Source: CAD feature listing. Evaluate the final solid. Frame: model axes, mm. Face numbers are marked on the shaded views. A direction names the side the tool comes from. Round coordinates to 2 decimals unless told otherwise and drop trailing zeros. Write each loop counter-clockwise with the first axis right and the second up, starting at its lowest first coordinate (ties: lowest second). Pieces come first, ordered by that corner, then holes. Notation, with made-up numbers: M -31.5,3.25 L 6.5,3.25 A13 cw 6.5,24.25 Z; hole C 8.5,25 d1. An arc over 180 degrees is marked long. Use a Markdown table: item, result.
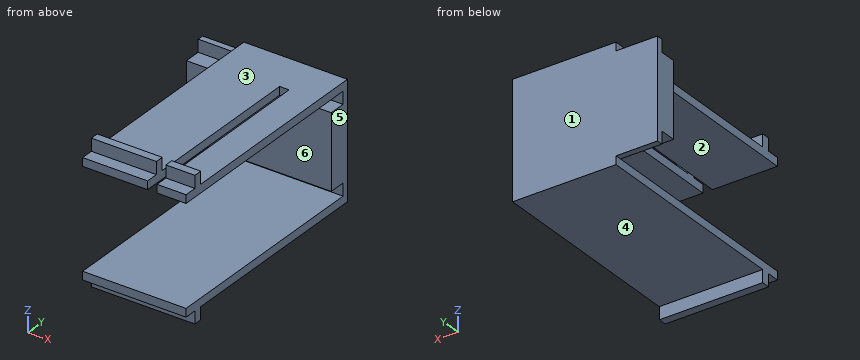
```python
from build123d import *

# Parameters (mm, degrees)
SKETCH1_W           = 25
SKETCH1_H           = 55
BOSS_EXTRUDE1_DEPTH = 2
SKETCH2_W           = 35
SKETCH2_H           = 1.5
BOSS_EXTRUDE2_DEPTH = 24
SKETCH3_W           = 25
SKETCH3_H           = 55
BOSS_EXTRUDE3_DEPTH = 2
SKETCH4_W           = 35
SKETCH4_H           = 18
BOSS_EXTRUDE4_DEPTH = 4
SKETCH5_W           = 2.3
SKETCH5_H           = 45
CUT_EXTRUDE1_DEPTH  = 2
SKETCH6_W           = 15.7
SKETCH6_H           = 2
SKETCH6_W_2         = 7
BOSS_EXTRUDE5_DEPTH = 3
SKETCH7_W           = 25
SKETCH7_H           = 2
BOSS_EXTRUDE6_DEPTH = 3


with BuildPart() as part:
    # Sketch1 → Boss-Extrude1 (new body)
    with BuildSketch(Plane.XY):
        Rectangle(SKETCH1_W, SKETCH1_H)
    extrude(amount=BOSS_EXTRUDE1_DEPTH)

    # Sketch2 → Boss-Extrude2 (add)
    with BuildSketch(Plane(origin=(0, 0, 0), x_dir=(-1, 0, 0), z_dir=(0, 0, -1))):
        with Locations((5, 26.75)):
            Rectangle(SKETCH2_W, SKETCH2_H)
    extrude(amount=BOSS_EXTRUDE2_DEPTH)

    # Sketch3 → Boss-Extrude3 (add)
    with BuildSketch(Plane(origin=(0, 0, -24), x_dir=(-1, 0, 0), z_dir=(0, 0, -1))):
        Rectangle(SKETCH3_W, SKETCH3_H)
    extrude(amount=BOSS_EXTRUDE3_DEPTH)

    # Sketch4 → Boss-Extrude4 (add)
    with BuildSketch(Plane.XZ.offset(-26)):
        with Locations((-5, -12)):
            Rectangle(SKETCH4_W, SKETCH4_H)
    extrude(amount=BOSS_EXTRUDE4_DEPTH)

    # Sketch5 → Cut-Extrude1 (cut)
    with BuildSketch(Plane.XY.offset(2)):
        with Locations((4.35, -5)):
            Rectangle(SKETCH5_W, SKETCH5_H)
    extrude(amount=-CUT_EXTRUDE1_DEPTH, mode=Mode.SUBTRACT)

    # Sketch6 → Boss-Extrude5 (add)
    with BuildSketch(Plane.XY.offset(2)):
        with Locations((-4.65, -23.5)):
            Rectangle(SKETCH6_W, SKETCH6_H)
        with Locations((9, -23.5)):
            Rectangle(SKETCH6_W_2, SKETCH6_H)
    extrude(amount=BOSS_EXTRUDE5_DEPTH)

    # Sketch7 → Boss-Extrude6 (add)
    with BuildSketch(Plane(origin=(0, 0, -26), x_dir=(-1, 0, 0), z_dir=(0, 0, -1))):
        with Locations((0, -23.5)):
            Rectangle(SKETCH7_W, SKETCH7_H)
    extrude(amount=BOSS_EXTRUDE6_DEPTH)


solid = part.part
```
Q1. Section B-B on x = -14. Return loops of the section in (y, z).
Results are:
| item | result |
|---|---|
| outline | M 22,-21 L 26,-21 L 26,-24 L 27.5,-24 L 27.5,0 L 26,0 L 26,-3 L 22,-3 Z |
Q2. Line query: L1, parallel to Z at x = -11.5, y = -6.5; L2, parallel to Z at x = -4, y = 23; L3, parallel to Z at x = -9.5, y = -23. Output: solid intervals per line, ascending.
Results are:
| item | result |
|---|---|
| L1 | -26 to -24, 0 to 2 |
| L2 | -26 to -24, -21 to -3, 0 to 2 |
| L3 | -29 to -24, 0 to 5 |
Q3. First-contact query: pin 1 Ø3 at (x, y) = (-12.5, 24) entering from -Z; pin 2 Ø3 at (x, z) = (-4, -20) entering from -Y; pin 3 Ø5.5 at (y, z) = (12.5, 3.5) entering from -X. Flat tips, straight axial feed; report the tip coordinate or a pass-through.
Results are:
| item | result |
|---|---|
| pin 1 | z = -26 |
| pin 2 | y = 22 |
| pin 3 | x = -12.5 |
Q4. Reachability of the marked faces 4, 5 and 6 from +Z, -Z, +X, -X, +Y, -Y: full face, straight path, thin tool, end or side. Return the list, or none.
Results are:
| item | result |
|---|---|
| face 4 | -Z, +X, -X, +Y |
| face 5 | +Z, -Z, +X, +Y, -Y |
| face 6 | +X, -X, -Y |
Q5. Section C-C on y = 24. Return loops of the section in (x, z), plus the area to 3 significant figures.
Results are:
| item | result |
|---|---|
| outline | M -22.5,-21 L 12.5,-21 L 12.5,-3 L -22.5,-3 Z; M -12.5,-26 L 12.5,-26 L 12.5,-24 L -12.5,-24 Z; M -12.5,0 L 12.5,0 L 12.5,2 L -12.5,2 Z |
| area | 730 mm^2 |
Q6. Section D-D on x = 10. Return loops of the section in (y, z), plus the area to 3 significant figures.
Results are:
| item | result |
|---|---|
| outline | M -27.5,-26 L -24.5,-26 L -24.5,-29 L -22.5,-29 L -22.5,-26 L 27.5,-26 L 27.5,2 L -22.5,2 L -22.5,5 L -24.5,5 L -24.5,2 L -27.5,2 L -27.5,0 L 26,0 L 26,-3 L 22,-3 L 22,-21 L 26,-21 L 26,-24 L -27.5,-24 Z |
| area | 340 mm^2 |
Q7. Mould query, pull axis Z, two halves, no side actions, for the marked faces 1, 2 and 3. Classes: +Z half, -Z half, draft (parallel to the pull), parting line (faces both ways), or undercut.
Results are:
| item | result |
|---|---|
| face 1 | draft |
| face 2 | undercut |
| face 3 | +Z half |
Q8. Section A-A on y = -14. Return loops of the section in (x, z), plus the area to 3 significant figures.
Results are:
| item | result |
|---|---|
| outline | M -12.5,-26 L 12.5,-26 L 12.5,-24 L -12.5,-24 Z; M -12.5,0 L 3.2,0 L 3.2,2 L -12.5,2 Z; M 5.5,0 L 12.5,0 L 12.5,2 L 5.5,2 Z |
| area | 95.4 mm^2 |
